from build123d import *

# Parameters (mm, degrees)
F0_W     = 241.3
F0_H     = 177.8
F0_R     = 34.925
F1_DEPTH = 9.525
F3_DEPTH = 19.05


with BuildPart() as f1:
    # F0 (on Front) → F1 (new body)
    with BuildSketch(Plane.XZ):
        Polygon((-177.8, 1168.4), (-342.9, 0), (342.9, 0), (177.8, 1168.4), align=None)
        with Locations((0, 809.869231)):
            Rectangle(F0_W, F0_H, mode=Mode.SUBTRACT)
        with Locations((0, 1013.069231)):
            Circle(F0_R, mode=Mode.SUBTRACT)
    extrude(amount=F1_DEPTH)

    # F2 (on face) → F3 (join)
    with BuildSketch(Plane(origin=(0, 0, 0), x_dir=(-1, 0, 0), z_dir=(0, 1, 0))):
        Polygon((-166.768402, 1155.7), (-358.675023, -202.408394), (-294.544206, -202.408394), (-265.94302, 0), (265.94302, 0), (294.544206, -202.408394), (358.675023, -202.408394), (166.768402, 1155.7), (111.610412, 1092.2), (256.970194, 63.5), (-256.970194, 63.5), (-111.610412, 1092.2), align=None)
        Polygon((166.768402, 1155.7), (-166.768402, 1155.7), (-111.610412, 1092.2), (111.610412, 1092.2), align=None)
    extrude(amount=F3_DEPTH)


solid = f1.part
Read the model definition and answer for the solid it produces. Units are mm, in the model's axes. A direction names the side the tool comes from. Give positions to 0.01 mm unless a question says otherwise; leave off trailing zeros. Loops run counter-clockwise (first coordinate to the right, second up) from the corner with the lowest first, then second, coordinate; pieces in that order, holes last. Notation, with made-up numbers: (68.25, 44.5) - (97.25, 44.5) arc R15 ccw to (97.25, 63.5) - close; hole circle Ø5 at (-10.75, 47). An arc over 180 degrees is marked (long way). Answer as CSV lines item,"result". Start each with the question number.
1) Each of these flat-tipped pins is pushed along its axis until it touches: pin 1 Ø2 at (y, z) = (8, 128) entering from +X; pin 2 Ø1.5 at (x, y) = (-279.5, -1.5) entering from -Z; pin 3 Ø3 at (y, z) = (-3.5, 988) entering from +X. Where does it stop, or does it pass through?
2) Find section C-C (x = 0). Write down the section's boundary in (y, z) (3 decimals).
3) Straight lines are drawn through the part: L1, parallel to Z at x = 0, y = -5; L2, parallel to Z at x = 83, y = 2.5; L3, parallel to Y at x = -137.5, z = 750 (3 decimals). For each, find the intervals that lie inside material, in ascending order. Write a range as from..to.
4) Find section D-D (z = 223). Write down the section's boundary in (x, y) (3 decimals).
5) Determine the mould class of faces 4 (the face through (16.116, -4.696, 982.085)), 5 (the face through (-264.065, 9.392, 467.139)), 6 (the face through (-211, 19.05, 430)) for opening direction X: released by +X, released by -X, zero draft, split by the parting line, or undercut.
6) Which of the six approach directions +Z, -Z, +X, -X, +Y, -Y give full straight-line access (tool end or side, diameter ignored) to faces 1 (the face through (-280.043, 9.392, -99.787)), 2 (the face through (261.38, 9.39, 486.15)), 3 (the face through (185.308, 9.392, 570.649))?
7) Find section A-A (y = 6.5). Write down the section's boundary in (x, z).
8) Find section B-B (z = 804). Write down the section's boundary in (x, y) (3 decimals).
Findings below:
1,pin 1,"x = 312.13"
1,pin 2,"z = 0"
1,pin 3,"x = 203.5"
2,outline,"(-9.525, 0) - (19.05, 0) - (19.05, 63.5) - (0, 63.5) - (0, 720.969) - (-9.525, 720.969) - close; (-9.525, 898.769) - (0, 898.769) - (0, 978.144) - (-9.525, 978.144) - close; (-9.525, 1047.994) - (0, 1047.994) - (0, 1092.2) - (19.05, 1092.2) - (19.05, 1155.7) - (0, 1155.7) - (0, 1168.4) - (-9.525, 1168.4) - close"
3,L1,"0..720.97, 898.77..978.14, 1047.99..1168.4"
3,L2,"0..63.5, 1092.2..1155.7"
3,L3,"-9.525..0"
4,outline,"(-311.389, -9.525) - (311.389, -9.525) - (311.389, 0) - (298.563, 0) - (298.563, 19.05) - (234.432, 19.05) - (234.432, 0) - (-234.432, 0) - (-234.432, 19.05) - (-298.563, 19.05) - (-298.563, 0) - (-311.389, 0) - close"
5,face 4,"undercut"
5,face 5,"released by -X"
5,face 6,"zero draft"
6,face 1,"-Z, +Y, -Y"
6,face 2,"+Z, +X, +Y"
6,face 3,"+Y"
7,outline,"(-358.68, -202.41) - (-294.54, -202.41) - (-265.94, 0) - (265.94, 0) - (294.54, -202.41) - (358.68, -202.41) - (166.77, 1155.7) - (-166.77, 1155.7) - close; hole (-256.97, 63.5) - (256.97, 63.5) - (111.61, 1092.2) - (-111.61, 1092.2) - close"
8,outline,"(-229.291, -9.525) - (-120.65, -9.525) - (-120.65, 0) - (-152.334, 0) - (-152.334, 19.05) - (-216.465, 19.05) - (-216.465, 0) - (-229.291, 0) - close; (120.65, -9.525) - (229.291, -9.525) - (229.291, 0) - (216.465, 0) - (216.465, 19.05) - (152.334, 19.05) - (152.334, 0) - (120.65, 0) - close"
